Study the drawing (mm; zero at the part's minimum x, y, z) and answer. A direction names the side the tool comes from. Give positions to 0.01 mm unless a question says otherwise; leave off trailing zeros. Order: outer loops, then holes, each group sorted by start corner. A loop starts at its lowest first (then second) coordinate and runs counter-clockwise, first axis right, second up. Notation, with made-up numbers: (-7.5, 46.25) - (45.5, 46.25) arc R24 ccw to (45.5, 82.25) - close; hole circle Ø4 at (37, 15). An arc over 180 degrees is marked (long way). Write each question's results on one line, items separated by ' | '. Start each with the question number.
Q1. Flat-ended cylindrical pins translate along their axes: P1, Ø10, axis at y = 69.5, z = 91.5, coming from the -X side; P2, Ø5, axis at y = 39, z = 11.5, coming from the +X side; P3, Ø10, axis at y = 69, z = 15, coming from the +X side; P4, Ø1, axis at x = 59.5, z = 13.5, coming from the -Y side. Find the tip coordinate at first contact, or state that the pin passes through.
Q2. For a pull along X with two mould halves and no side action, classify the marked faces 1, 2 and 3 as +X half, -X half, draft (parallel to the pull), parting line (faces both ways), or undercut.
Q3. Find section B-B on z = 10. Give the vertices of the cut face in (x, y).
Q4. Find section A-A on y = 59.5. Give the vertices of the cut face in (x, z), and give its area (3 significant figures).
Q5. Find the intervals of material crossed by line 1 along Z through (x, y) = (70, 48.5); line 2 along X through (y, z) = (52.5, 35) (1 decimal); line 3 along X through (y, z) = (72, 64), in increasing order. Write a range as from..to.
Q6. Find section C-C on z = 48. Give the vertices of the cut face in (x, y).
Q7. Find section D-D on x = 26.5. Give the vertices of the cut face in (y, z).
Q8. A tool of negligible diameter and unlimited length cuts with its end or side. For the marked faces 4 and 5, from which of +Z, -Z, +X, -X, +Y, -Y can it reach the whole face along a straight path? Write none if from no direction.
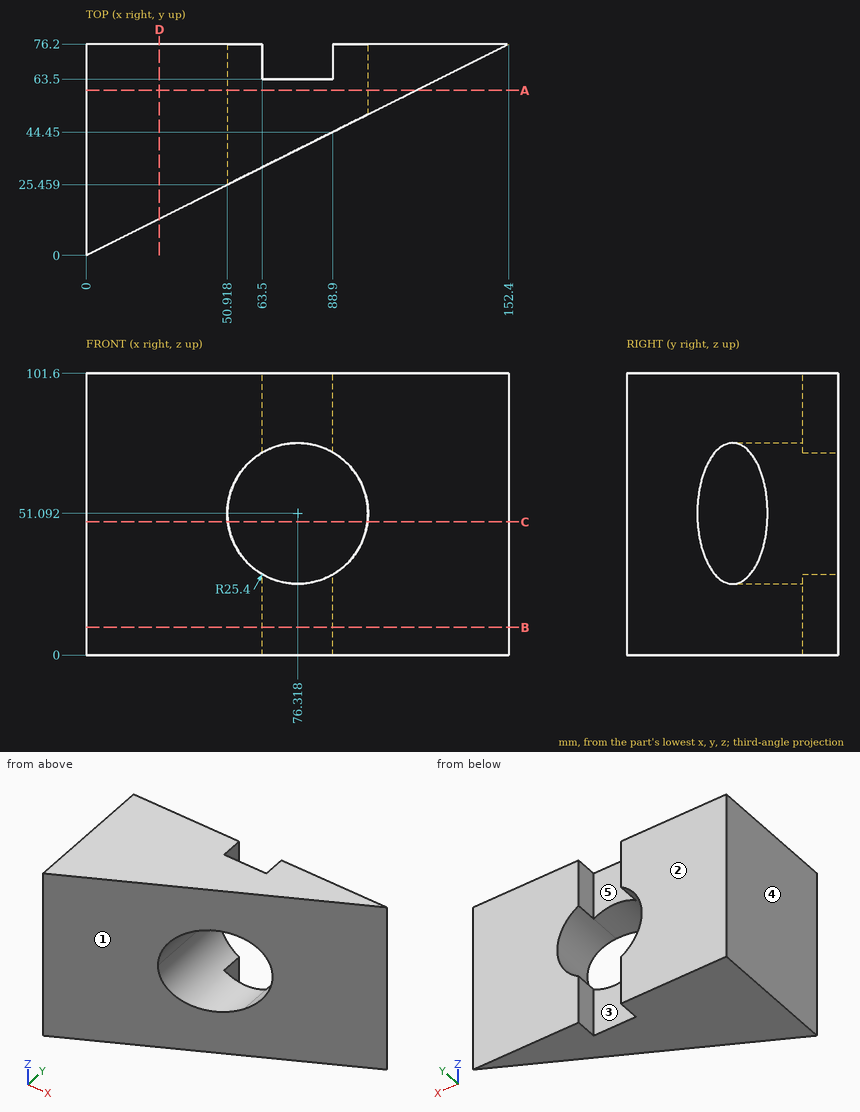
Working result:
1) P1: x = 0 | P2: x = 83 | P3: x = 148 | P4: y = 29.5
2) face 1: +X half | face 2: draft | face 3: undercut
3) outline: (0, 0) - (152.4, 76.2) - (88.9, 76.2) - (88.9, 63.5) - (63.5, 63.5) - (63.5, 76.2) - (0, 76.2) - close
4) outline: (0, 0) - (119, 0) - (119, 101.6) - (0, 101.6) - close; hole circle Ø50.8 at (76.32, 51.09) | area: 10,100 mm²
5) line 1: 0..26.49, 75.69..101.6 | line 2: 0..56.7, 96..105 | line 3: 0..54.44, 98.19..144
6) outline: (0, 0) - (51.11, 25.55) - (51.11, 76.2) - (0, 76.2) - close; (101.53, 50.76) - (152.4, 76.2) - (101.53, 76.2) - close
7) outline: (13.25, 0) - (76.2, 0) - (76.2, 101.6) - (13.25, 101.6) - close
8) face 4: +Z, -Z, -X, +Y, -Y | face 5: +Z, -Z, +Y
